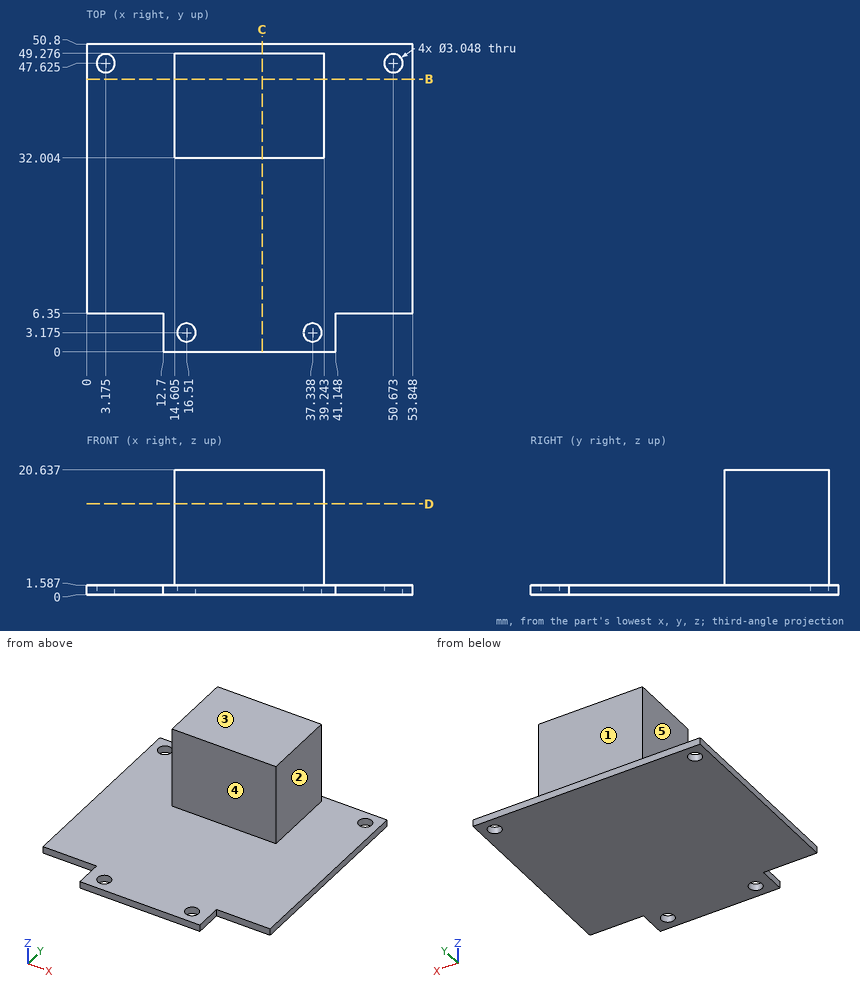
Verification items for this drawing (mm, ordinates from the low corner). A direction names the side the tool comes from. Round coordinates to 2 decimals unless told otherwise and drop trailing zeros. Order: outer loops, then holes, each group sorted by start corner. A loop starts at its lowest first (then second) coordinate and runs counter-clockwise, first axis right, second up. Notation, with made-up numbers: M 30.5,6 L 85.5,6 A23 ccw 85.5,15 Z; hole C 38.5,66.25 d7. An arc over 180 degrees is marked long. Answer in a Markdown table with one row per item. Add a question column.
Item 1: Depth check by flat-ended pin: pin 1 Ø0.8 at (y, z) = (2, 1) entering from +X; pin 2 Ø5 at (y, z) = (40, 10.5) entering from -X (1 decimal); pin 3 Ø9.5 at (x, z) = (27.5, 13) entering from -Y. Enter the tip coordinate at first touch or a pass-through.
Item 2: Sectioned sample at B-B, the plane y = 45. Enter the section's corners in (x, z) (1 decimal), plus the area to 3 significant figures.
Item 3: Sectioned sample at D-D, the plane z = 15. Enter the section's corners in (x, y) (1 decimal).
Item 4: Set-up check for the marked faces 1, 2, 3, 4 and 5: record each of +Z, -Z, +X, -X, +Y, -Y from which the full face is reachable in a straight line by a thin tool's end or side.
Item 5: Material ranges on L1, parallel to Y at x = 16.51, z = 0.45; L2, parallel to Z at x = 7.5, y = 11; L3, parallel to X at y = 33, z = 5.75 (1 decimal), recorded low to high. Write a range as [from, to].
Item 6: Sectioned sample at C-C, the plane x = 29. Enter the section's corners in (y, z) (1 decimal), plus the area to 3 significant figures.
Filled in:
| question | item | result |
|---|---|---|
| 1 | pin 1 | stops at x = 41.15 |
| 1 | pin 2 | stops at x = 14.6 |
| 1 | pin 3 | stops at y = 32 |
| 2 | outline | M 0,0 L 53.8,0 L 53.8,1.6 L 39.2,1.6 L 39.2,20.6 L 14.6,20.6 L 14.6,1.6 L 0,1.6 Z |
| 2 | area | 555 mm² |
| 3 | outline | M 14.6,32 L 39.2,32 L 39.2,49.3 L 14.6,49.3 Z |
| 4 | face 1 | +Z, +X, -X, +Y |
| 4 | face 2 | +Z, +X, +Y, -Y |
| 4 | face 3 | +Z, +X, -X, +Y, -Y |
| 4 | face 4 | +Z, +X, -X, -Y |
| 4 | face 5 | +Z, -X, +Y, -Y |
| 5 | L1 | y = [0, 1.65], [4.7, 50.8] |
| 5 | L2 | z = [0, 1.59] |
| 5 | L3 | x = [14.6, 39.2] |
| 6 | outline | M 0,0 L 50.8,0 L 50.8,1.6 L 49.3,1.6 L 49.3,20.6 L 32,20.6 L 32,1.6 L 0,1.6 Z |
| 6 | area | 410 mm² |
